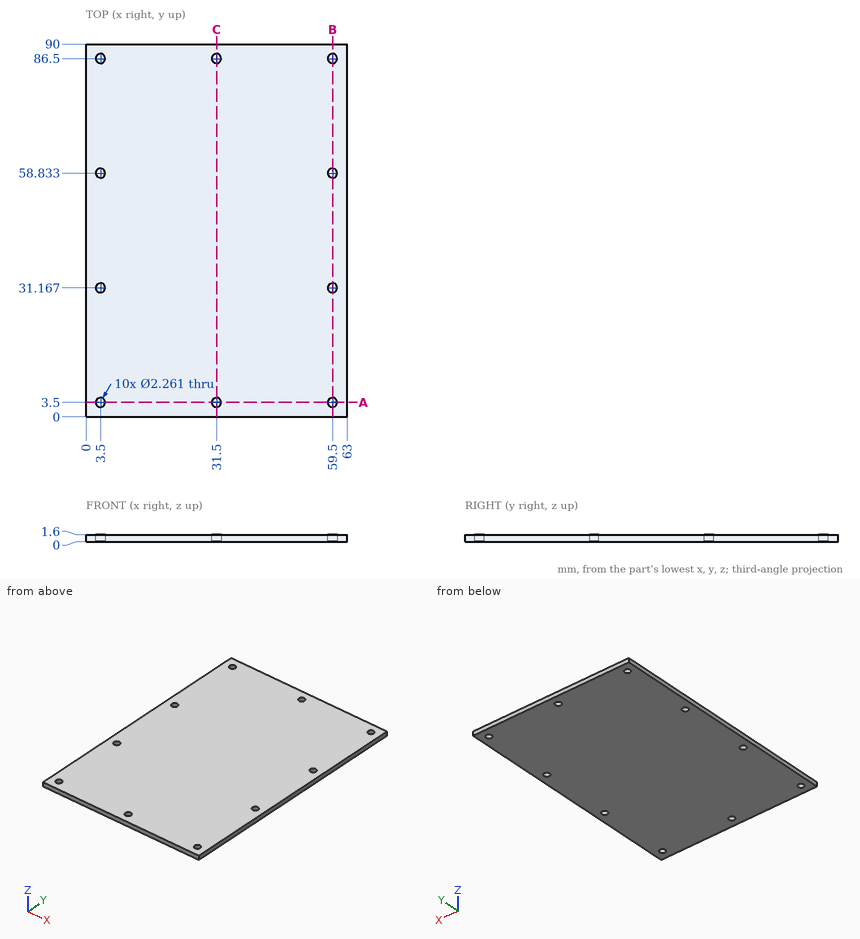
Verification items for this drawing (mm, ordinates from the low corner). Coordinates: 2 decimals unless noted, no trailing zeros. Order: outer loops, then holes, each group sorted by start corner. A loop starts at its lowest first (then second) coordinate and runs counter-clockwise, first axis right, second up. Notation, with made-up numbers: M 47.5,87.25 L 84.5,87.25 A33 ccw 84.5,118.25 Z; hole C 2,-15.5 d9. An arc over 180 degrees is marked long. Answer as a JSON object with one key per item and string values.
Q1. Cross-section at B-B on x = 59.5. Record the cut outline in (y, z).
Results are:
{"outline": "M 0,0 L 2.37,0 L 2.37,1.6 L 0,1.6 Z; M 4.63,0 L 30.04,0 L 30.04,1.6 L 4.63,1.6 Z; M 32.3,0 L 57.7,0 L 57.7,1.6 L 32.3,1.6 Z; M 59.96,0 L 85.37,0 L 85.37,1.6 L 59.96,1.6 Z; M 87.63,0 L 90,0 L 90,1.6 L 87.63,1.6 Z"}
Q2. Cross-section at C-C on x = 31.5. Record the cut outline in (y, z).
Results are:
{"outline": "M 0,0 L 2.37,0 L 2.37,1.6 L 0,1.6 Z; M 4.63,0 L 85.37,0 L 85.37,1.6 L 4.63,1.6 Z; M 87.63,0 L 90,0 L 90,1.6 L 87.63,1.6 Z"}
Q3. Cross-section at A-A on y = 3.5. Record the cut outline in (x, z).
Results are:
{"outline": "M 0,0 L 2.37,0 L 2.37,1.6 L 0,1.6 Z; M 4.63,0 L 30.37,0 L 30.37,1.6 L 4.63,1.6 Z; M 32.63,0 L 58.37,0 L 58.37,1.6 L 32.63,1.6 Z; M 60.63,0 L 63,0 L 63,1.6 L 60.63,1.6 Z"}
Q4. Scan lines: line 1 (X direction, y = 59, z = 0.85); line 2 (Y direction, x = 3.5, z = 0.5); line 3 (X direction, y = 86.5, z = 0.95). Record each from-to range of solid material in increasing order.
Results are:
{"line 1": "x = 0 to 2.38, 4.62 to 58.38, 60.62 to 63", "line 2": "y = 0 to 2.37, 4.63 to 30.04, 32.3 to 57.7, 59.96 to 85.37, 87.63 to 90", "line 3": "x = 0 to 2.37, 4.63 to 30.37, 32.63 to 58.37, 60.63 to 63"}
